Source: CAD feature listing. Evaluate the final solid. Frame: model axes, mm. A direction names the side the tool comes from. Give positions to 0.01 mm unless a question says otherwise; leave off trailing zeros. Write each loop counter-clockwise with the first axis right and the second up, starting at its lowest first coordinate (ties: lowest second). Pieces come first, ordered by that corner, then holes.
```python
from build123d import *

# Parameters (mm, degrees)
F0_W     = 40
F0_H     = 34
F1_DEPTH = 26.5
F3_DEPTH = 34.001
F5_DEPTH = 27


with BuildPart() as f1:
    # F0 (on Front) → F1 (new body, symmetric)
    with BuildSketch(Plane.XZ):
        Rectangle(F0_W, F0_H)
    extrude(amount=F1_DEPTH, both=True)

    # F2 (on face) → F3 (cut, through all)
    with BuildSketch(Plane.XY.offset(17)):
        with BuildLine():
            Line((-12.5, -26.5), (12.5, -26.5))
            ThreePointArc((12.5, -26.5), (0, -14), (-12.5, -26.5))
        make_face()
    extrude(amount=-F3_DEPTH, mode=Mode.SUBTRACT)

    # F4 (on face) → F5 (cut)
    with BuildSketch(Plane(origin=(0, 26.5, 0), x_dir=(-1, 0, 0), z_dir=(0, 1, 0))):
        with BuildLine():
            Line((20, 17), (-7, 17))
            ThreePointArc((-7, 17), (0.908116908, -2.091883092), (20, -10))
            Line((20, -10), (20, 17))
        make_face()
    extrude(amount=-F5_DEPTH, mode=Mode.SUBTRACT)


solid = f1.part
```
1. Line query: L1, parallel to X at y = -22.5, z = -7; L2, parallel to Y at x = -15, z = 4; L3, parallel to Y at x = 3, z = -9.5. Output: solid intervals per line, ascending.
2. Cut plane C-C, the plane y = 7. Return the cut outline in (x, z).
3. Cut plane B-B, the plane z = 4. Return the cut outline in (x, y).
4. Cut plane D-D, the plane x = -14.5. Return the cut outline in (y, z), then the cut area to 3 significant figures.
5. Access query for faces 1 (the cylindrical face through (-0.7, 13.19, -1.88)), 2 (the cylindrical face through (0, -14, 0)). Directions: +Z, -Z, +X, -X, +Y, -Y. A direction counts if a zero-diameter tool reaches every point of the face in a straight line with its end or side. Return the directions, or none.
6. Cut plane A-A, the plane y = -19. Return the cut outline in (x, z), then the cut area to 3 significant figures.
7. Contact query for flat-ended pins moving along their axis: P1, Ø2, axis at x = -5.5, z = 4.5, coming from the -Y side; P2, Ø1.5, axis at x = 8, z = 12, coming from the -Y side; P3, Ø1, axis at x = -12.5, y = 17, coming from the +Z side. Output: stop coordinate, or through.
Response values:
1. L1: x = -20 to -11.84, 11.84 to 20
1. L2: y = -26.5 to -0.5
1. L3: y = -14.37 to 26.5
2. outline: (-20, -17) - (20, -17) - (20, 17) - (7, 17) arc R27 cw to (-20, -10) - close
3. outline: (-20, -26.5) - (-12.5, -26.5) arc R12.5 cw to (12.5, -26.5) - (20, -26.5) - (20, 26.5) - (3.66, 26.5) - (3.66, -0.5) - (-20, -0.5) - close
4. outline: (-26.5, -17) - (26.5, -17) - (26.5, -9.43) - (-0.5, -9.43) - (-0.5, 17) - (-26.5, 17) - close
4. area: 1,090 mm2
5. face 1: +Z, -X, +Y
5. face 2: +Z, -Z, -Y
6. outline: (-20, -17) - (-10, -17) - (-10, 17) - (-20, 17) - close; (10, -17) - (20, -17) - (20, 17) - (10, 17) - close
6. area: 680 mm2
7. P1: stops at y = -15.82
7. P2: stops at y = -17.57
7. P3: stops at z = -8.79
